For this review, take the finished solid that the model builds, in its own axes (mm). A direction names the side the tool comes from. Give positions to 0.01 mm unless a question says otherwise; leave off trailing zeros. Write each loop counter-clockwise with the first axis right and the second up, starting at its lowest first coordinate (ties: lowest second). Pieces come first, ordered by that corner, then holes. Notation, with made-up numbers: M -15.5,-10.75 L 26.5,-10.75 A9 cw 26.5,-2.75 Z; hole C -30.5,37.25 d1. An arc over 180 degrees is marked long. Use one line per item in the form item = value. Start each with the question number.
Q1. Tool access review of faces 1 (the flat face through (-9, 62, -9)), 2 (the flat face through (-11, 80, -4)), 3 (the cylindrical face through (11.923, 73.01, 3.755)): name each direction out of +Z, -Z, +X, -X, +Y, -Y from which nothing blocks a thin tool from reaching the whole face with its end or side.
Q2. For probe 1 along Z at (x, y) = (0.5, 27.5); probe 2 along X at (y, z) = (58, -6.5); probe 3 along Z at (x, y) = (-9.5, 56), list the stretches that pass through material, from the lowest coordinate up. Write a range as [from, to].
Q3. Consider section B-B on z = 0. Write out the cut boundary in (x, y), and give its area (3 significant figures).
Q4. Consider section D-D on y = 74.5. Write out the cut boundary in (x, z).
Q5. Consider section A-A on x = 0. Write out the cut boundary in (y, z).
Q6. Mouldability with a two-part tool opening along Z and no side actions: class faces 4 (the cylindrical face through (10.78, 40.56, 3.39)), 5 (the flat face through (6, 0, -10)), 6 (the cylindrical face through (11.923, 63.824, 3.755)) as released by +Z, released by -Z, zero draft, split by the parting line, or undercut.
Q7. Consider section C-C on y = 47.5. Write out the cut boundary in (x, z), and give its area (3 significant figures).
Q8. Clearance check with flat-ended pins moving along their axes: pin 1 Ø4 at (y, z) = (65, 7.5) entering from +X; pin 2 Ø3 at (y, z) = (36, 3) entering from -X; pin 3 Ø3 at (x, y) = (9.5, 58.5) entering from +Z; pin 4 Ø10 at (x, y) = (-4.5, 17.5) entering from +Z. State where each tip first meets the part, or that it passes through.
```python
from build123d import *

# Parameters (mm, degrees)
FILLET1_R = 0.5


with BuildPart() as part:
    # Sketch1 → Revolve1 (revolve)
    with BuildSketch(Plane.XY):
        with BuildLine():
            Line((11.3, 0), (11.3, 80))
            Line((11.3, 80), (12.5, 80))
            Line((12.5, 80), (12.5, 66.7))
            ThreePointArc((12.5, 66.7), (13, 66.2), (12.5, 65.7))
            Line((12.5, 65.7), (12.5, 62))
            Line((12.5, 62), (13.5, 62))
            Line((13.5, 62), (13.5, 0))
            Line((13.5, 0), (11.3, 0))
        make_face()
    revolve(axis=Axis((0, 52.2625, 0), (0, -1, 0)))

    # Fillet1
    fillet1_edges = [part.edges().sort_by_distance(p)[0] for p in [
        (-12.5, 80, 0),
    ]]
    fillet(fillet1_edges, radius=FILLET1_R)


solid = part.part
```
Working result:
q1.face_1 = none
q1.face_2 = +Z, -Z, +X, -X, +Y
q1.face_3 = +Y
q2.probe_1 = [-13.49, -11.29], [11.29, 13.49]
q2.probe_2 = [-11.83, -9.24], [9.24, 11.83]
q2.probe_3 = [-9.59, -6.12], [6.12, 9.59]
q3.outline = M -13.5,0 L -11.3,0 L -11.3,80 L -12,80 A0.5 ccw -12.5,79.5 L -12.5,66.7 A0.5 ccw -12.5,65.7 L -12.5,62 L -13.5,62 Z; M 11.3,0 L 13.5,0 L 13.5,62 L 12.5,62 L 12.5,65.7 A0.5 ccw 12.5,66.7 L 12.5,79.5 A0.5 ccw 12,80 L 11.3,80 Z
q3.area = 317 mm²
q4.outline = C 0,0 d25; hole C 0,0 d22.6
q5.outline = M 0,-13.5 L 62,-13.5 L 62,-12.5 L 65.7,-12.5 A0.5 ccw 66.7,-12.5 L 79.5,-12.5 A0.5 ccw 80,-12 L 80,-11.3 L 0,-11.3 Z; M 0,11.3 L 80,11.3 L 80,12 A0.5 ccw 79.5,12.5 L 66.7,12.5 A0.5 ccw 65.7,12.5 L 62,12.5 L 62,13.5 L 0,13.5 Z
q6.face_4 = undercut
q6.face_5 = zero draft
q6.face_6 = split by the parting line
q7.outline = C 0,0 d27; hole C 0,0 d22.6
q7.area = 171 mm²
q8.pin_1 = 11.61
q8.pin_2 = -13.42
q8.pin_3 = 10.87
q8.pin_4 = 13.5
